For this review, take the finished solid that the model builds, in its own axes (mm). Coordinates: 2 decimals unless noted, no trailing zeros. Loops run counter-clockwise (first coordinate to the right, second up) from the corner with the lowest first, then second, coordinate; pieces in that order, holes last. Notation, with made-up numbers: (-13, 4) - (13, 4) arc R22 cw to (13, 39) - close; hole circle Ø10 at (76, 63). An arc over 180 degrees is marked (long way). One line per item, written item: value. Start each with the question number.
1. Insertion check: pin 1 (1.2 mm diameter, centred on y = 1.5, z = 82.5, fed in from -X); pin 2 (1.5 mm diameter, centred on x = 126, y = 1.5, fed in from -Z); pin 3 (1.2 mm diameter, centred on y = 2.5, z = 83.5, fed in from +X). Each pin has a flat end and moves straight along its axis. Give the tip position at first contact, or say it passes through.
2. To check wall thickness, follow line 1 (X direction, y = 2.2, z = 0); line 2 (X direction, y = 1.3, z = 9); line 3 (Z direction, x = 42, y = 1.3). State the ranges of each line that lie inside material, in increasing order. Write a range as from..to.
3. Take a section at B-B, the plane y = 1.5. State the section outline as (x, z) points, and give its area (3 significant figures).
4. Take a section at A-A, the plane z = 0. State the section outline as (x, y) points, and give its area (3 significant figures).
5. Take a section at C-C, the plane x = 0. State the section outline as (y, z) points, and give its area (3 significant figures).
```python
from build123d import *

# Parameters (mm, degrees)
SKETCH_4_R      = 50
EXTRUDE_3_DEPTH = 4


with BuildPart() as part:
    # 草图4 → 凸台-拉伸3 (new body)
    with BuildSketch(Plane(origin=(0, 0, 0), x_dir=(1, 0, 0), z_dir=(0, 1, 0))):
        Polygon((-125, 75), (-125, 90), (125, 90), (125, 75), (128, 75), (128, -75), (125, -75), (125, -90), (-125, -90), (-125, -75), (-128, -75), (-128, 75), align=None)
        with Locations(Location((0, 0, 0), (0, 0, 270))):
            Circle(SKETCH_4_R, mode=Mode.SUBTRACT)
    extrude(amount=EXTRUDE_3_DEPTH)


solid = part.part
```
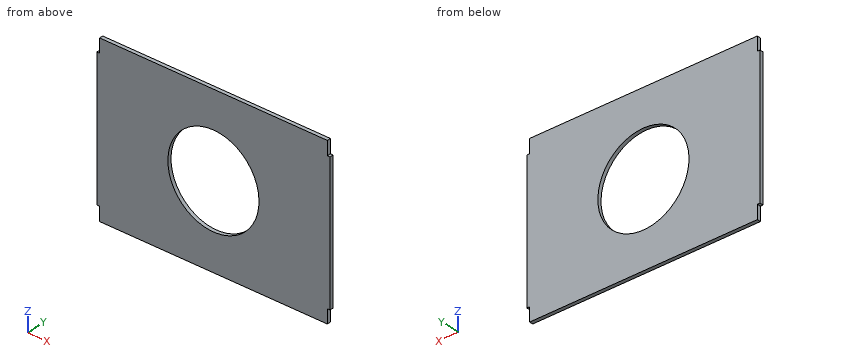
Solutions:
1. pin 1: x = -125
1. pin 2: z = -75
1. pin 3: x = 125
2. line 1: -128..-50, 50..128
2. line 2: -128..-49.18, 49.18..128
2. line 3: -90..-27.13, 27.13..90
3. outline: (-128, -75) - (-125, -75) - (-125, -90) - (125, -90) - (125, -75) - (128, -75) - (128, 75) - (125, 75) - (125, 90) - (-125, 90) - (-125, 75) - (-128, 75) - close; hole circle Ø100 at (0, 0)
3. area: 38,000 mm2
4. outline: (-128, 0) - (-50, 0) - (-50, 4) - (-128, 4) - close; (50, 0) - (128, 0) - (128, 4) - (50, 4) - close
4. area: 624 mm2
5. outline: (0, -90) - (4, -90) - (4, -50) - (0, -50) - close; (0, 50) - (4, 50) - (4, 90) - (0, 90) - close
5. area: 320 mm2
